Model file for the job. Use its own axes, mm. A direction names the side the tool comes from. Round coordinates to 2 decimals unless told otherwise and drop trailing zeros. Loops run counter-clockwise (first coordinate to the right, second up) from the corner with the lowest first, then second, coordinate; pieces in that order, holes last. Notation, with made-up numbers: (-5.5, -21) - (31.5, -21) arc R28 cw to (31.5, 10) - close; hole circle Ø7 at (19, 76). An arc over 180 degrees is marked (long way). Use one line per item in the form item = value.
from build123d import *

# Parameters (mm, degrees)
SKETCH1_R           = 2
BOSS_EXTRUDE1_DEPTH = 13
CUT_EXTRUDE2_DEPTH  = 9
CUT_EXTRUDE3_DEPTH  = 9
SKETCH7_R           = 0.5
CUT_EXTRUDE4_DEPTH  = 4


with BuildPart() as part:
    # Sketch1 → Boss-Extrude1 (new body)
    with BuildSketch(Plane.XY):
        Polygon((-96, 0), (-54.120862841, 0), (-54.120862841, 5), (-47, 5), (-47, 14.5), (-47, 35), (-51, 35), (-56, 35), (-56, 31), (-51, 31), (-51, 14.5), (-59, 14.5), (-59, 10.5), (-84, 10.5), (-84, 14.5), (-96, 14.5), align=None)
        with Locations((-87.5, 8.5)):
            Circle(SKETCH1_R, mode=Mode.SUBTRACT)
        with Locations((-55.5, 8.5)):
            Circle(SKETCH1_R, mode=Mode.SUBTRACT)
    extrude(amount=BOSS_EXTRUDE1_DEPTH)

    # Sketch5 → Cut-Extrude2 (cut)
    with BuildSketch(Plane.XY.offset(13)):
        Polygon((-84, 14.5), (-96, 14.5), (-96, 0), (-54.120862841, 0), (-54.120862841, 5), (-51, 5), (-51, 14.5), (-59, 14.5), (-59, 10.5), (-84, 10.5), align=None)
    extrude(amount=-CUT_EXTRUDE2_DEPTH, mode=Mode.SUBTRACT)

    # Sketch6 → Cut-Extrude3 (cut)
    with BuildSketch(Plane(origin=(0, 0, 0), x_dir=(-1, 0, 0), z_dir=(0, 0, -1))):
        Polygon((51, 31), (56, 31), (56, 35), (47, 35), (47, 14.5), (51, 14.5), align=None)
    extrude(amount=-CUT_EXTRUDE3_DEPTH, mode=Mode.SUBTRACT)

    # Sketch7 → Cut-Extrude4 (cut)
    with BuildSketch(Plane(origin=(0, 31, 0), x_dir=(-1, 0, 0), z_dir=(0, -1, 0))):
        with Locations((53.5, -11)):
            Circle(SKETCH7_R)
    extrude(amount=-CUT_EXTRUDE4_DEPTH, mode=Mode.SUBTRACT)


solid = part.part
1. Pull direction X, two halves, no side cores. Call faces 6 (the cylindrical face through (-56.974, 9.852, 1.972)), 7 (the flat face through (-54.1, 31, 11.4)), 8 (the flat face through (-51, 15.3, 9.4)): +X half, -X half, draft (parallel to the pull), parting line (faces both ways), or undercut.
Geometry check:
face_6 = undercut
face_7 = draft
face_8 = -X half
2. Tool access for faces 1 (the flat face through (-59, 13, 2)), 2 (the flat face through (-74, 6, 4)), 3 (the flat face through (-52, 14.5, 3)), 4 (the flat face through (-54.121, 2, 2)), 5 (the cylindrical face through (-53, 33, 11)): list every direction of +Z, -Z, +X, -X, +Y, -Y with a clear straight run to the whole face (end or side of a thin tool).
Geometry check:
face_1 = +Z, -Z, +Y
face_2 = +Z, -X, +Y, -Y
face_3 = -Z, +X, -X, +Y
face_4 = +Z, -Z, +X, -Y
face_5 = +Y, -Y
3. Cut at B-B, the plane y = 8.5. Give the cut face in (x, z), plus the area to 3 significant figures.
Geometry check:
outline = (-96, 0) - (-89.5, 0) - (-89.5, 4) - (-96, 4) - close; (-85.5, 0) - (-57.5, 0) - (-57.5, 4) - (-85.5, 4) - close; (-53.5, 0) - (-47, 0) - (-47, 13) - (-51, 13) - (-51, 4) - (-53.5, 4) - close
area = 200 mm^2
4. Flat gauge pins, fed straight in: pin 1 (2 mm diameter, centred on x = -79.5, y = 4.5, fed in from +Z); pin 2 (2 mm diameter, centred on x = -75.5, z = 1.5, fed in from +Y); pin 3 (5.5 mm diameter, centred on x = -51.5, z = 5.5, fed in from -Y); pin 4 (5 mm diameter, centred on y = 16, z = 7, fed in from +X). Where does each tip first touch, or does it go through?
Geometry check:
pin_1 = 4
pin_2 = 10.5
pin_3 = 5
pin_4 = -47
5. Wall check: probe 1 along X at (y, z) = (8.5, 2.2); probe 2 along Y at (x, z) = (-87.5, 1.05); probe 3 along X at (y, z) = (33.25, 11). Give the ranges that are in metal, low to high.
Geometry check:
probe_1 = -96 to -89.5, -85.5 to -57.5, -53.5 to -47
probe_2 = 0 to 6.5, 10.5 to 14.5
probe_3 = -56 to -54, -53 to -47
6. Cut at A-A, the plane z = 11. Give the cut face in (x, y).
Geometry check:
outline = (-56, 31) - (-54, 31) - (-54, 35) - (-56, 35) - close; (-53, 31) - (-51, 31) - (-51, 5) - (-47, 5) - (-47, 35) - (-53, 35) - close
7. Cut at D-D, the plane x = -55.5. Give the cut face in (y, z), plus the area to 3 significant figures.
Geometry check:
outline = (0, 0) - (6.5, 0) - (6.5, 4) - (0, 4) - close; (10.5, 0) - (14.5, 0) - (14.5, 4) - (10.5, 4) - close; (31, 9) - (35, 9) - (35, 13) - (31, 13) - close
area = 58.0 mm^2
8. Cut at C-C, the plane y = 13. Give the cut face in (x, z).
Geometry check:
outline = (-96, 0) - (-84, 0) - (-84, 4) - (-96, 4) - close; (-59, 0) - (-47, 0) - (-47, 13) - (-51, 13) - (-51, 4) - (-59, 4) - close
